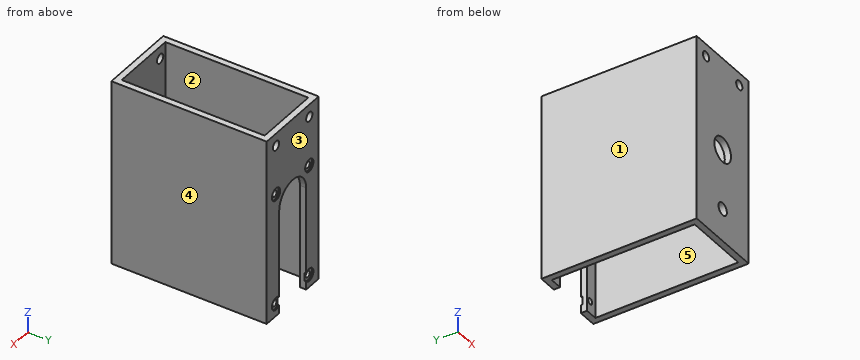
Autodesk Inventor part; units mm, degrees
ref_plane "YZ Plane" through (0, 0, 0) normal (1, 0, 0) x (0, 1, 0)
ref_plane "XZ Plane" through (0, 0, 0) normal (0, 1, 0) x (-1, 0, 0)
ref_plane "XY Plane" through (0, 0, 0) normal (0, 0, 1) x (1, 0, 0)
sketch "スケッチ1" plane through (0, 0, 0) normal (0, 0, 1) x (1, 0, 0)
  line L0 (-12.5, 25) -> (12.5, 25)
  line L1 (12.5, 25) -> (12.5, -25)
  line L2 (12.5, -25) -> (-12.5, -25)
  line L3 (-12.5, -25) -> (-12.5, 25)
  line L4 (-10.5, 23) -> (10.5, 23)
  line L5 (10.5, 23) -> (10.5, -23)
  line L6 (10.5, -23) -> (-10.5, -23)
  line L7 (-10.5, -23) -> (-10.5, 23)
  point P0 (0, 0)
  dimension "d0" = 25
  dimension "d1" = 50
  dimension "d2" = 46
  dimension "d3" = 21
  dimension "d4" = 25
  dimension "d5" = 23
  dimension "d6" = 10.5
  dimension "d7" = 12.5
extrude "押し出し1" add sketch "スケッチ1" along normal blind 60
sketch "スケッチ2" plane through (-12.5, 25, 0) normal (0, 1, 0) x (1, 0, 0)
  line L0 (0, 0) -> (25, 0)
  line L1 (0, 0) -> (0, -60)
  arc A0 (6, -33.5) -> (19, -33.5) centre (12.5, -33.5) ccw
  line L2 (6, -33.5) -> (6, 0)
  line L3 (19, -33.5) -> (19, 0)
  point P0 (12.5, 0)
  dimension "d10" = 13
  dimension "d11" = 33.5
  dimension "d12" = 12.5
extrude "押し出し2" cut sketch "スケッチ2" against normal blind 2
sketch "スケッチ3" plane through (-12.5, 25, 60) normal (0, 1, 0) x (1, 0, 0)
  arc A0 (6, 26.5) -> (19, 26.5) centre (12.5, 26.5) ccw
  circle A1 centre (4.5, 20) radius 1
  circle A2 centre (4.5, 56) radius 1
  circle A3 centre (20.5, 56) radius 1
  circle A4 centre (20.5, 20) radius 1
  point P0 (12.5, 60)
  dimension "d15" = 6.5
  dimension "d16" = 6.5
  dimension "d17" = 2
  dimension "d18" = 8
  dimension "d19" = 8
  dimension "d20" = 8
  dimension "d21" = 8
  dimension "d22" = 29.5
  dimension "d23" = 29.5
hole "穴1" at (-8, 25, 4) at (8, 25, 4) at (8, 25, 40) at (-8, 25, 40) direction (0, -1, 0) diameter 2 depth 2 tip angle 118 counterbore diameter 4 counterbore depth 0.5
sketch "スケッチ4" plane through (-12.5, -25, 0) normal (0, -1, 0) x (1, 0, 0)
  line L0 (25, 0) -> (0, 0)
  line L1 (25, 0) -> (25, 60)
  circle A0 centre (12.5, 10.5) radius 2
  point P0 (12.5, 0)
  dimension "d31" = 4
  dimension "d32" = 12.5
  dimension "d33" = 10.5
hole "穴2" at (0, -25, 10.5) direction (0, 1, 0) diameter 4 end through all
sketch "スケッチ5" plane through (-12.5, 25, 60) normal (0, 1, 0) x (1, 0, 0)
  line L0 (0, 0) -> (25, 0)
  arc A0 (6, 26.5) -> (19, 26.5) centre (12.5, 26.5) ccw
  circle A1 centre (20.5, 4) radius 1.5
  circle A2 centre (4.5, 4) radius 1.5
  point P0 (12.5, 60)
  dimension "d43" = 4
  dimension "d44" = 4
  dimension "d46" = 8
  dimension "d47" = 8
  dimension "d57" = 3
hole "穴4" at (-8, 25, 56) at (8, 25, 56) direction (0, -1, 0) diameter 3 end through all
thread "ねじ1"
thread "ねじ2"
thread "ねじ3"
thread "ねじ4"
sketch "スケッチ7" plane through (-12.5, -25, 0) normal (0, -1, 0) x (1, 0, 0)
  line L0 (25, 60) -> (0, 60)
  line L1 (25, 0) -> (25, 60)
  circle A0 centre (12.5, 30) radius 4
  point P0 (12.5, 0)
  dimension "d78" = 30
  dimension "d79" = 8
  dimension "d80" = 12.5
hole "穴5" at (0, -25, 30) direction (0, 1, 0) diameter 8 end through all
properties part number "07" material "アルミニウム 6061"
Source: CAD feature listing. Evaluate the final solid. Frame: model axes, mm. Face numbers are marked on the shaded views. A direction names the side the tool comes from. Round coordinates to 2 decimals unless told otherwise and drop trailing zeros. Order: outer loops, then holes, each group sorted by start corner. A loop starts at its lowest first (then second) coordinate and runs counter-clockwise, first axis right, second up. Notation, with made-up numbers: (42, 79.5) -> (62, 79.5) arc R18 ccw to (62, 105.5) -> close; hole circle Ø5 at (-16, 9). An arc over 180 degrees is marked (long way). One line per item, written item: value. Start each with the question number.
Q1. Draft query along X for the marked faces 1, 2 and 3. Return one class per face: pulls with the +X half, pulls with the -X half, needs draft (parallel to the pull), parting line crosses it, or undercut.
Q2. Section query D-D (z = 30). Return the cut outline in (x, y), plus the area to 3 significant figures.
Q3. Material intervals for probe 1 along X at (y, z) = (23.6, 4); probe 2 along X at (y, z) = (-23.4, 56); probe 3 along Z at (x, y) = (8, 24.7), sorted ascending.
Q4. Pin query (flat end, axial travel): pin 1 (1.8 mm diameter, centred on x = 8, z = 40, fed in from +Y); pin 2 (4.5 mm diameter, centred on x = 9, z = 40, fed in from +Y); pin 3 (6.5 mm diameter, centred on x = 0, z = 30, fed in from +Y). Return the tip coordinate at first contact, or that it passes through.
Q5. Access query for the marked faces 4 and 5. Directions: +Z, -Z, +X, -X, +Y, -Y. A direction counts if a zero-diameter tool reaches every point of the face in a straight line with its end or side. Return the directions, or none.
Q6. Section query A-A (z = 4). Return the cut outline in (x, y), plus the area to 4 significant figures.
Q7. Section query C-C (y = -0.5). Return the cut outline in (x, z), plus the area to 3 significant figures.
Q8. Section query B-B (x = 8). Give the number of separate pieces and of enclosed holes in the cut face, plus the area to 3 significant figures.
Findings below:
1. face 1: pulls with the -X half
1. face 2: undercut
1. face 3: needs draft
2. outline: (-12.5, -25) -> (-4, -25) -> (-4, -23) -> (-10.5, -23) -> (-10.5, 23) -> (-6.5, 23) -> (-6.5, 25) -> (-12.5, 25) -> close; (4, -25) -> (12.5, -25) -> (12.5, 25) -> (6.5, 25) -> (6.5, 23) -> (10.5, 23) -> (10.5, -23) -> (4, -23) -> close
2. area: 242 mm²
3. probe 1: -12.5 to -9, -7 to -6.5, 6.5 to 7, 9 to 12.5
3. probe 2: -12.5 to -9.5, -6.5 to 6.5, 9.5 to 12.5
3. probe 3: 0 to 2, 6 to 38, 42 to 54.5, 57.5 to 60
4. pin 1: y = -23
4. pin 2: y = 25
4. pin 3: through
5. face 4: +Z, -Z, +X, +Y, -Y
5. face 5: +Z, -Z
6. outline: (-12.5, -25) -> (12.5, -25) -> (12.5, 25) -> (10, 25) -> (10, 24.5) -> (9, 24.5) -> (9, 23) -> (10.5, 23) -> (10.5, -23) -> (-10.5, -23) -> (-10.5, 23) -> (-9, 23) -> (-9, 24.5) -> (-10, 24.5) -> (-10, 25) -> (-12.5, 25) -> close; (-7, 23) -> (-6.5, 23) -> (-6.5, 24.5) -> (-7, 24.5) -> close; (6.5, 23) -> (7, 23) -> (7, 24.5) -> (6.5, 24.5) -> close
6. area: 248.5 mm²
7. outline: (-12.5, 0) -> (-10.5, 0) -> (-10.5, 60) -> (-12.5, 60) -> close; (10.5, 0) -> (12.5, 0) -> (12.5, 60) -> (10.5, 60) -> close
7. area: 240 mm²
8. separate pieces: 6
8. enclosed holes: 0
8. area: 218 mm²
